Geometry check sheet. Reference: drawing and pictorial views, mm from the part's lowest x, y, z. Round coordinates to 2 decimals unless told otherwise and drop trailing zeros. Order: outer loops, then holes, each group sorted by start corner. A loop starts at its lowest first (then second) coordinate and runs counter-clockwise, first axis right, second up.
(1) Sectioned sample at D-D (x = 26). Record the boundary of the cut face in (y, z).
(2) Sectioned sample at B-B (z = 5). Record the boundary of the cut face in (x, y).
(3) Material ranges on line 1 along X through (y, z) = (0.8, 5); line 2 along X through (y, z) = (2.4, 30.5); line 3 along Z through (x, y) = (45.5, 2.35), recorded low to high.
(4) Sectioned sample at C-C (y = 1.9). Give the number of separate pieces and of enclosed holes in the cut face, plus the area to 3 significant figures.
(5) Sectioned sample at A-A (x = 75). Record the boundary of the cut face in (y, z), plus the area to 3 significant figures.
(6) Go/stop test with a flat-tipped pin: pin 1 (17 mm diameter, centred on x = 25, z = 25, fed in from -Y). Record where the tip stops, or that it passes through.
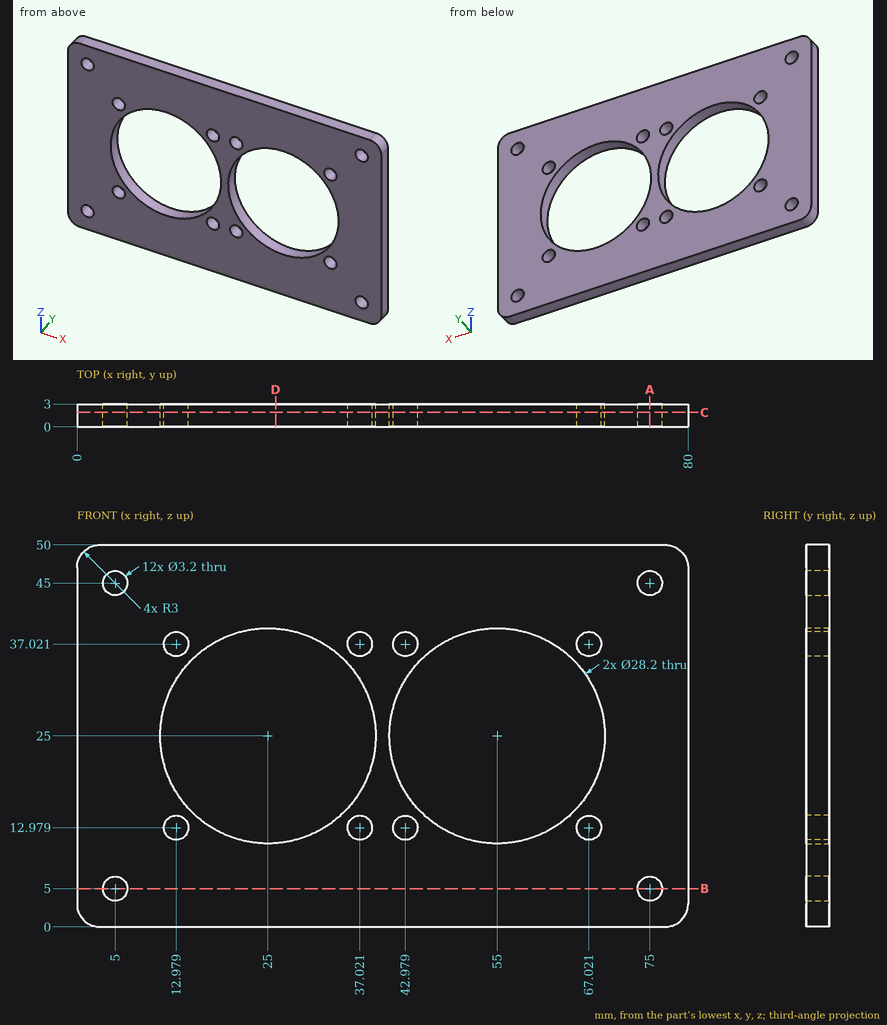
Answer below:
1. outline: (0, 0) - (3, 0) - (3, 10.94) - (0, 10.94) - close; (0, 39.06) - (3, 39.06) - (3, 50) - (0, 50) - close
2. outline: (0, 0) - (3.4, 0) - (3.4, 3) - (0, 3) - close; (6.6, 0) - (73.4, 0) - (73.4, 3) - (6.6, 3) - close; (76.6, 0) - (80, 0) - (80, 3) - (76.6, 3) - close
3. line 1: x = 0 to 3.4, 6.6 to 73.4, 76.6 to 80
3. line 2: x = 0 to 12.02, 37.98 to 42.02, 67.98 to 80
3. line 3: z = 0 to 14.58, 35.42 to 50
4. separate pieces: 1
4. enclosed holes: 14
4. area: 2,650 mm2
5. outline: (0, 0) - (3, 0) - (3, 3.4) - (0, 3.4) - close; (0, 6.6) - (3, 6.6) - (3, 43.4) - (0, 43.4) - close; (0, 46.6) - (3, 46.6) - (3, 50) - (0, 50) - close
5. area: 131 mm2
6. pin 1: passes through
